CAD build for the part. Positions are in the model's coordinates, mm. Face numbers are marked on the shaded views. A direction names the side the tool comes from. Round coordinates to 2 decimals unless told otherwise and drop trailing zeros. Write each loop counter-clockwise with the first axis right and the second up, starting at its lowest first coordinate (ties: lowest second). Pieces come first, ordered by that corner, then holes. Notation, with made-up numbers: (60, 42) - (103, 42) arc R17 ccw to (103, 73) - close; hole circle Ø6 at (67, 79.25). An arc over 180 degrees is marked (long way). Put each result on its own line as item: value. Start each with the question number.
Item 1: Cut at C-C (x = 75). Give the cut face in (y, z).
Item 2: Mould opens along X. For the marked faces 1, 2 and 3 say: released by +X, released by -X, zero draft, split by the parting line, or undercut.
Item 3: Pin check, flat tips, straight feed: pin 1 Ø1 at (x, z) = (2, -2) entering from +Y; pin 2 Ø3 at (x, z) = (34.5, -57.5) entering from -Y; pin 3 Ø12 at (x, z) = (72, -19) entering from +Y. Stop position of each tip, or through.
Item 4: Cut at B-B (y = 8). Give the cut face in (x, z).
Item 5: 3-axis set-ups, long thin cutter, end or side, ignore diameter. For the marked faces 4, 5 and 6: which of +Z, -Z, +X, -X, +Y, -Y reach the whole face in a straight line?
Item 6: Drill centre lines: line 1 (Z direction, x = 34.5, y = 5.5); line 2 (X direction, y = 10.5, z = -51.5); line 3 (Z direction, x = 108.5, y = 33.6). Where is each one in solid material? Low to high. Write a range as from..to.
Item 7: Cut at D-D (z = -40). Give the cut face in (x, y).
Item 8: Cut at A-A (z = -6.5). Give the cut face in (x, y), and give its area (3 significant figures).
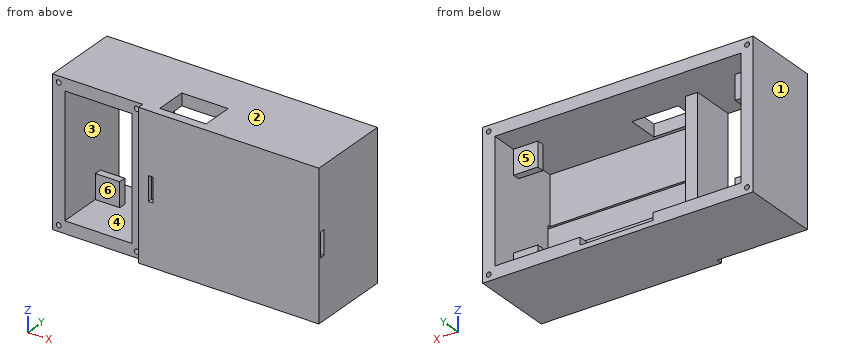
```python
from build123d import *

# Parameters (mm, degrees)
SKETCH1_W           = 111
SKETCH1_H           = 60
BOSS_EXTRUDE1_DEPTH = 34.5
SKETCH2_W           = 101
SKETCH2_H           = 50
CUT_EXTRUDE1_DEPTH  = 11
CUT_EXTRUDE3_DEPTH  = 14
CUT_EXTRUDE5_START  = -2
SKETCH5_W           = 27.5
SKETCH5_H           = 50
SKETCH5_W_2         = 68.5
CUT_EXTRUDE5_DEPTH  = 18.5
SKETCH6_W           = 37
SKETCH6_H           = 60
CUT_EXTRUDE6_DEPTH  = 2.5
SKETCH7_R           = 1
CUT_EXTRUDE7_DEPTH  = 4
SKETCH8_R           = 1
CUT_EXTRUDE8_DEPTH  = 4
SKETCH9_W           = 19
SKETCH9_H           = 13
CUT_EXTRUDE9_DEPTH  = 10
SKETCH10_W          = 10
SKETCH10_H          = 2
CUT_EXTRUDE10_DEPTH = 70
SKETCH11_W          = 2
SKETCH11_H          = 10
CUT_EXTRUDE11_DEPTH = 2
SKETCH12_W          = 30
SKETCH12_H          = 3
CUT_EXTRUDE12_DEPTH = 32.5


with BuildPart() as part:
    # Sketch1 → Boss-Extrude1 (new body)
    with BuildSketch(Plane(origin=(0, 0, 0), x_dir=(1, 0, 0), z_dir=(0, 1, 0))):
        with Locations((55.5, 30)):
            Rectangle(SKETCH1_W, SKETCH1_H)
    extrude(amount=BOSS_EXTRUDE1_DEPTH)

    # Sketch2 → Cut-Extrude1 (cut)
    with BuildSketch(Plane(origin=(0, 34.5, 0), x_dir=(1, 0, 0), z_dir=(0, 1, 0))):
        with Locations((55.5, 30)):
            Rectangle(SKETCH2_W, SKETCH2_H)
    extrude(amount=-CUT_EXTRUDE1_DEPTH, mode=Mode.SUBTRACT)

    # Sketch3 → Cut-Extrude3 (cut)
    with BuildSketch(Plane(origin=(0, 34.5, 0), x_dir=(1, 0, 0), z_dir=(0, 1, 0))):
        Polygon((5, 45), (15, 45), (15, 55), (96, 55), (96, 45), (106, 45), (106, 15), (96, 15), (96, 5), (15, 5), (15, 15), (5, 15), align=None)
    extrude(amount=-CUT_EXTRUDE3_DEPTH, mode=Mode.SUBTRACT)

    # Sketch5 → Cut-Extrude5 (cut)
    with BuildSketch(Plane.XZ.offset(CUT_EXTRUDE5_START)):
        with Locations((18.75, -30)):
            Rectangle(SKETCH5_W, SKETCH5_H)
        with Locations((71.75, -30)):
            Rectangle(SKETCH5_W_2, SKETCH5_H)
    extrude(amount=-CUT_EXTRUDE5_DEPTH, mode=Mode.SUBTRACT)

    # Sketch6 → Cut-Extrude6 (cut)
    with BuildSketch(Plane.XZ):
        with Locations((18.5, -30)):
            Rectangle(SKETCH6_W, SKETCH6_H)
    extrude(amount=-CUT_EXTRUDE6_DEPTH, mode=Mode.SUBTRACT)

    # Sketch7 → Cut-Extrude7 (cut)
    with BuildSketch(Plane(origin=(0, 2.5, 0), x_dir=(-1, 0, 0), z_dir=(0, -1, 0))):
        with Locations((-2.5, 57.5)):
            Circle(SKETCH7_R)
        with Locations((-34.5, 57.5)):
            Circle(SKETCH7_R)
        with Locations((-34.5, 2.5)):
            Circle(SKETCH7_R)
        with Locations((-2.5, 2.5)):
            Circle(SKETCH7_R)
    extrude(amount=-CUT_EXTRUDE7_DEPTH, mode=Mode.SUBTRACT)

    # Sketch8 → Cut-Extrude8 (cut)
    with BuildSketch(Plane(origin=(0, 34.5, 0), x_dir=(1, 0, 0), z_dir=(0, 1, 0))):
        with Locations((2.5, 57.5)):
            Circle(SKETCH8_R)
        with Locations((108.5, 57.5)):
            Circle(SKETCH8_R)
        with Locations((108.5, 2.360383006)):
            Circle(SKETCH8_R)
        with Locations((2.5, 2.5)):
            Circle(SKETCH8_R)
    extrude(amount=-CUT_EXTRUDE8_DEPTH, mode=Mode.SUBTRACT)

    # Sketch9 → Cut-Extrude9 (cut)
    with BuildSketch(Plane.XY):
        with Locations((52.792502494, 10)):
            Rectangle(SKETCH9_W, SKETCH9_H)
    extrude(amount=-CUT_EXTRUDE9_DEPTH, mode=Mode.SUBTRACT)

    # Sketch10 → Cut-Extrude10 (cut)
    with BuildSketch(Plane(origin=(111, 0, 0), x_dir=(0, 0, -1), z_dir=(1, 0, 0))):
        with Locations((30, 2)):
            Rectangle(SKETCH10_W, SKETCH10_H)
    extrude(amount=-CUT_EXTRUDE10_DEPTH, mode=Mode.SUBTRACT)

    # Sketch11 → Cut-Extrude11 (cut, through all)
    with BuildSketch(Plane(origin=(0, 1, 0), x_dir=(1, 0, 0), z_dir=(0, 1, 0))):
        with Locations((42, 30)):
            Rectangle(SKETCH11_W, SKETCH11_H)
    extrude(amount=-CUT_EXTRUDE11_DEPTH, mode=Mode.SUBTRACT)

    # Sketch12 → Cut-Extrude12 (cut)
    with BuildSketch(Plane(origin=(0, 34.5, 0), x_dir=(1, 0, 0), z_dir=(0, 1, 0))):
        with Locations((56, 56.5)):
            Rectangle(SKETCH12_W, SKETCH12_H)
    extrude(amount=-CUT_EXTRUDE12_DEPTH, mode=Mode.SUBTRACT)


solid = part.part
```
Output values:
1. outline: (0, -60) - (34.5, -60) - (34.5, -55) - (2, -55) - (2, -35) - (1, -35) - (1, -25) - (2, -25) - (2, -5) - (34.5, -5) - (34.5, 0) - (0, 0) - close
2. face 1: released by -X
2. face 2: zero draft
2. face 3: undercut
3. pin 1: y = 34.5
3. pin 2: y = 2.5
3. pin 3: y = 2
4. outline: (0, -60) - (111, -60) - (111, 0) - (62.29, 0) - (62.29, -5) - (106, -5) - (106, -55) - (71, -55) - (71, -58) - (41, -58) - (41, -55) - (37.5, -55) - (37.5, -5) - (43.29, -5) - (43.29, 0) - (0, 0) - close; hole (5, -55) - (32.5, -55) - (32.5, -5) - (5, -5) - close
5. face 4: none
5. face 5: +Y
5. face 6: -Y
6. line 1: -60..-58.5, -56.5..-3.5, -1.5..0
6. line 2: 0..5, 32.5..37.5, 106..111
6. line 3: -60..-58.5, -56.5..-3.36, -1.36..0
7. outline: (0, 2.5) - (5, 2.5) - (5, 34.5) - (0, 34.5) - close; (32.5, 2.5) - (37, 2.5) - (37, 0) - (111, 0) - (111, 34.5) - (106, 34.5) - (106, 2) - (37.5, 2) - (37.5, 20.5) - (32.5, 20.5) - close
8. outline: (0, 2.5) - (5, 2.5) - (5, 20.5) - (15, 20.5) - (15, 23.5) - (5, 23.5) - (5, 34.5) - (0, 34.5) - close; (32.5, 2.5) - (37, 2.5) - (37, 0) - (111, 0) - (111, 34.5) - (106, 34.5) - (106, 23.5) - (96, 23.5) - (96, 20.5) - (106, 20.5) - (106, 2) - (37.5, 2) - (37.5, 20.5) - (32.5, 20.5) - close
8. area: 621 mm2
